Geometry: final body of the model. Coordinates: model frame, mm. Give positions to 0.01 mm unless a question says otherwise; leave off trailing zeros. Write each loop counter-clockwise with the first axis right and the second up, starting at its lowest first coordinate (ties: lowest second). Pieces come first, ordered by that corner, then holes. Notation, with made-up numbers: (56, 11) -> (74, 11) arc R19 ccw to (74, 32) -> close; hole circle Ø1 at (58, 72). An arc over 180 degrees is marked (long way). Use CSV: the item, a comma, the result in double quotes. Start each with the question number.
1) Section B-B (z = 6.35). Output: boundary loops of the cut face in (x, y), plus the area to 3 significant figures.
2) Draft query along Z for faces 1 (the face through (-2.766, -3.863, 5.175)), 2 (the face through (-19, -4, 12.7)), 3 (the face through (-36.651, -3.863, 1.528)). Return one class per face: pulls with the +Z half, pulls with the -Z half, needs draft (parallel to the pull), parting line crosses it, or undercut.
3) Section C-C (z = 8). Output: boundary loops of the cut face in (x, y), plus the area to 3 significant figures.
4) Section D-D (z = 1). Output: boundary loops of the cut face in (x, y).
5) Contact query for flat-ended pins moving along their axis: P1, Ø1.5, axis at y = -5, z = 9.5, coming from the +X side; P2, Ø2, axis at y = -3, z = 1.5, coming from the -X side; P3, Ø3.5, axis at x = -5.6, z = 6.35, coming from the -Y side. Output: stop coordinate, or through.
6) Material intervals for line 1 (X direction, y = -3.5, z = 7.25); line 2 (Z direction, x = -5, y = -1.75); line 3 (X direction, y = -2.5, z = 9), sorted ascending. Write a range as [from, to].
7) Section A-A (y = -1). Output: boundary loops of the cut face in (x, z).
```python
from build123d import *

# Parameters (mm, degrees)
F0_W     = 38.1
F0_H     = 12.7
F1_DEPTH = 7.62
F2_R     = 3.068034
F3_DEPTH = 7.621
F4_R     = 5.08


with BuildPart() as f1:
    # F0 (on Front) → F1 (new body)
    with BuildSketch(Plane.XZ):
        with Locations((-19.05, 6.35)):
            Rectangle(F0_W, F0_H)
    extrude(amount=F1_DEPTH)

    # F2 (on face) → F3 (cut, through all)
    with BuildSketch(Plane.XZ.offset(7.62)):
        with Locations((-5.599708, 6.35)):
            Circle(F2_R)
    extrude(amount=-F3_DEPTH, mode=Mode.SUBTRACT)

    # F4
    f4_edges = [f1.edges().sort_by_distance(p)[0] for p in [
        (0, -3.81, 12.7),
        (0, -3.81, 0),
        (-38.1, -3.81, 12.7),
        (-38.1, -3.81, 0),
    ]]
    fillet(f4_edges, radius=F4_R)


solid = f1.part
```
Answers follow:
1,outline,"(-38.1, -7.62) -> (-8.67, -7.62) -> (-8.67, 0) -> (-38.1, 0) -> close; (-2.53, -7.62) -> (0, -7.62) -> (0, 0) -> (-2.53, 0) -> close"
1,area,"244 mm^2"
2,face 1,"undercut"
2,face 2,"pulls with the +Z half"
2,face 3,"pulls with the -Z half"
3,outline,"(-38.09, -7.62) -> (-8.19, -7.62) -> (-8.19, 0) -> (-38.09, 0) -> close; (-3.01, -7.62) -> (-0.01, -7.62) -> (-0.01, 0) -> (-3.01, 0) -> close"
3,area,"251 mm^2"
4,outline,"(-36.05, -7.62) -> (-2.05, -7.62) -> (-2.05, 0) -> (-36.05, 0) -> close"
5,P1,"stops at x = -0.13"
5,P2,"stops at x = -37.4"
5,P3,"passes through"
6,line 1,"x = [-38.1, -8.53], [-2.67, 0]"
6,line 2,"z = [0, 3.34], [9.36, 12.7]"
6,line 3,"x = [-37.91, -7.15], [-4.05, -0.19]"
7,outline,"(-38.1, 5.08) arc R5.08 ccw to (-33.02, 0) -> (-5.08, 0) arc R5.08 ccw to (0, 5.08) -> (0, 7.62) arc R5.08 ccw to (-5.08, 12.7) -> (-33.02, 12.7) arc R5.08 ccw to (-38.1, 7.62) -> close; hole circle Ø6.14 at (-5.6, 6.35)"
